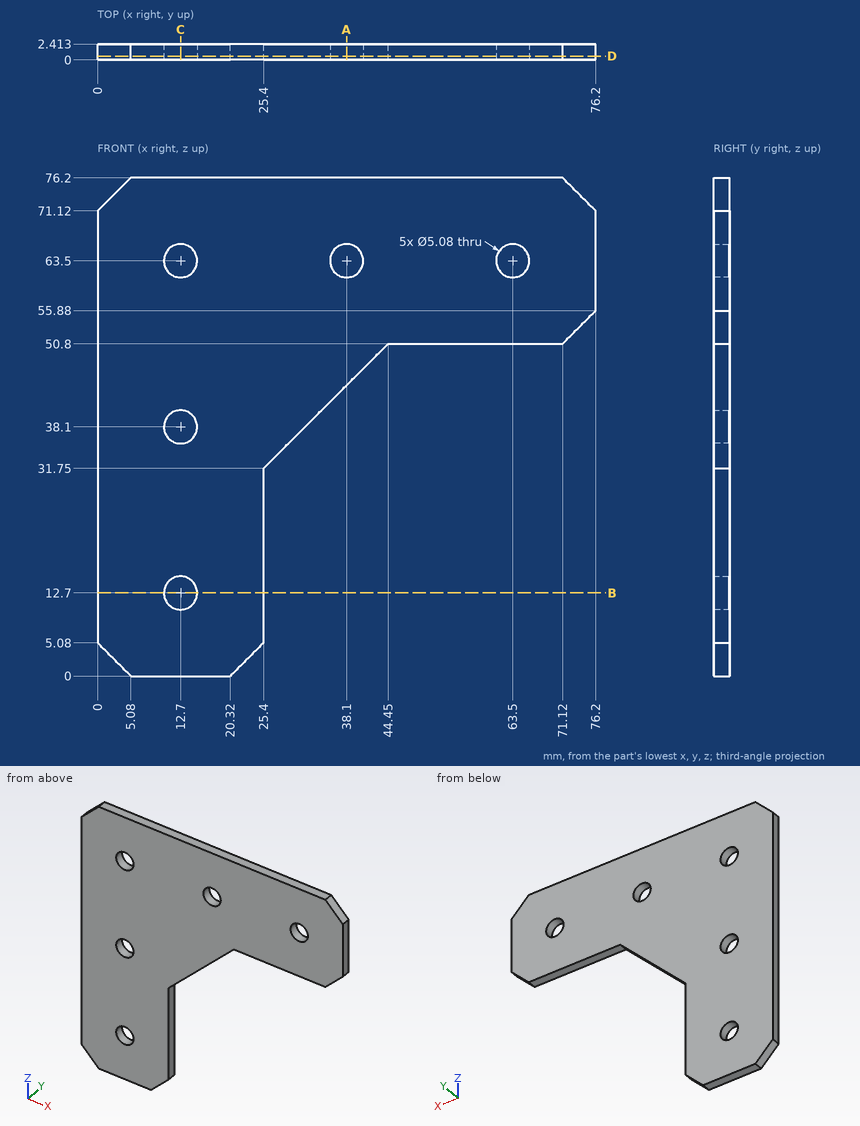
Could you check a few things on this drawing? It's one solid part, dimensions in mm from its lowest x, y, z. Coordinates: 2 decimals unless noted, no trailing zeros. Write each loop counter-clockwise with the first axis right and the second up, starting at its lowest first coordinate (ties: lowest second). Pieces come first, ordered by that corner, then holes. Notation, with made-up numbers: (76, 2.25) - (93, 2.25) arc R23 ccw to (93, 32.25) - close; hole circle Ø2 at (-7, 0). An arc over 180 degrees is marked (long way). Use one line per item in the form item = value.
1) Suppose I cut it at A-A, the plane x = 38.1. Write out the boundary of the cut face in (y, z).
Solved:
outline = (0, 44.45) - (2.41, 44.45) - (2.41, 60.96) - (0, 60.96) - close; (0, 66.04) - (2.41, 66.04) - (2.41, 76.2) - (0, 76.2) - close
2) I'm going to push a flat-ended pin straight in: P1, Ø4, axis at x = 63.5, z = 63.5, coming from the -Y side. Where does the tip first touch, or does it pass through?
Solved:
P1 = through
3) Suppose I cut it at C-C, the plane x = 12.7. Write out the boundary of the cut face in (y, z), plus the area to 3 significant figures.
Solved:
outline = (0, 0) - (2.41, 0) - (2.41, 10.16) - (0, 10.16) - close; (0, 15.24) - (2.41, 15.24) - (2.41, 35.56) - (0, 35.56) - close; (0, 40.64) - (2.41, 40.64) - (2.41, 60.96) - (0, 60.96) - close; (0, 66.04) - (2.41, 66.04) - (2.41, 76.2) - (0, 76.2) - close
area = 147 mm2
4) Suppose I cut it at D-D, the plane y = 0.55. Write out the boundary of the cut face in (x, z).
Solved:
outline = (0, 5.08) - (5.08, 0) - (20.32, 0) - (25.4, 5.08) - (25.4, 31.75) - (44.45, 50.8) - (71.12, 50.8) - (76.2, 55.88) - (76.2, 71.12) - (71.12, 76.2) - (5.08, 76.2) - (0, 71.12) - close; hole circle Ø5.08 at (12.7, 12.7); hole circle Ø5.08 at (12.7, 38.1); hole circle Ø5.08 at (12.7, 63.5); hole circle Ø5.08 at (38.1, 63.5); hole circle Ø5.08 at (63.5, 63.5)
5) Suppose I cut it at B-B, the plane z = 12.7. Write out the boundary of the cut face in (x, y), plus the area to 3 significant figures.
Solved:
outline = (0, 0) - (10.16, 0) - (10.16, 2.41) - (0, 2.41) - close; (15.24, 0) - (25.4, 0) - (25.4, 2.41) - (15.24, 2.41) - close
area = 49.0 mm2
6) I need wall thicknesses on line 1 (X direction, y = 1.7, z = 63.5); line 2 (X direction, y = 1.05, z = 12.7); line 3 (X direction, y = 2.2, z = 12). Which ranges of each line are inside material? Lowest first, please.
Solved:
line_1 = 0 to 10.16, 15.24 to 35.56, 40.64 to 60.96, 66.04 to 76.2
line_2 = 0 to 10.16, 15.24 to 25.4
line_3 = 0 to 10.26, 15.14 to 25.4
